Verification items for this drawing (mm, ordinates from the low corner). A direction names the side the tool comes from. Coordinates: 2 decimals unless noted, no trailing zeros. Order: outer loops, then holes, each group sorted by start corner. A loop starts at its lowest first (then second) coordinate and runs counter-clockwise, first axis right, second up. Notation, with made-up numbers: (-23, -17) -> (29, -17) arc R20 cw to (29, -10) -> close; hole circle Ø10 at (62.5, 56). An arc over 180 degrees is marked (long way). Write item = value, one per line. Start each with the question number.
1. Cross-section at B-B on x = 13.5. Record the cut outline in (y, z).
2. Release check for a two-part mould opening along X. For the marked faces 1, 2 and 3 record: +X half, -X half, draft (parallel to the pull), parting line (faces both ways), or undercut.
3. Set-up check for the marked faces 4 and 5: record each of +Z, -Z, +X, -X, +Y, -Y from which the full face is reachable in a straight line by a thin tool's end or side.
4. Cross-section at A-A on z = 60. Record the cut outline in (x, y), plus the area to 3 significant figures.
5. Cross-section at C-C on y = 55.5. Record the cut outline in (x, z), plus the area to 3 significant figures.
6. Thickness scan on line 1 along X through (y, z) = (53.5, 53.5); line 2 along Z through (x, y) = (68, 52); line 3 along Z through (x, y) = (12.5, 24). Record the ranges inside material, lowest first. Write a range as from..to.
7. Cross-section at D-D on z = 51. Record the cut outline in (x, y), plus the area to 3 significant figures.
8. Go/stop test with flat-tipped pins: P1, Ø1, axis at x = 78, z = 47.5, coming from the -Y side; P2, Ø5, axis at x = 14, y = 19.5, coming from the -Z side; P3, Ø9, axis at x = 43, y = 45.5, coming from the +Z side; P4, Ø1.5, axis at x = 23, y = 38, coming from the +Z side. Record where each tip stops, or that it passes through.
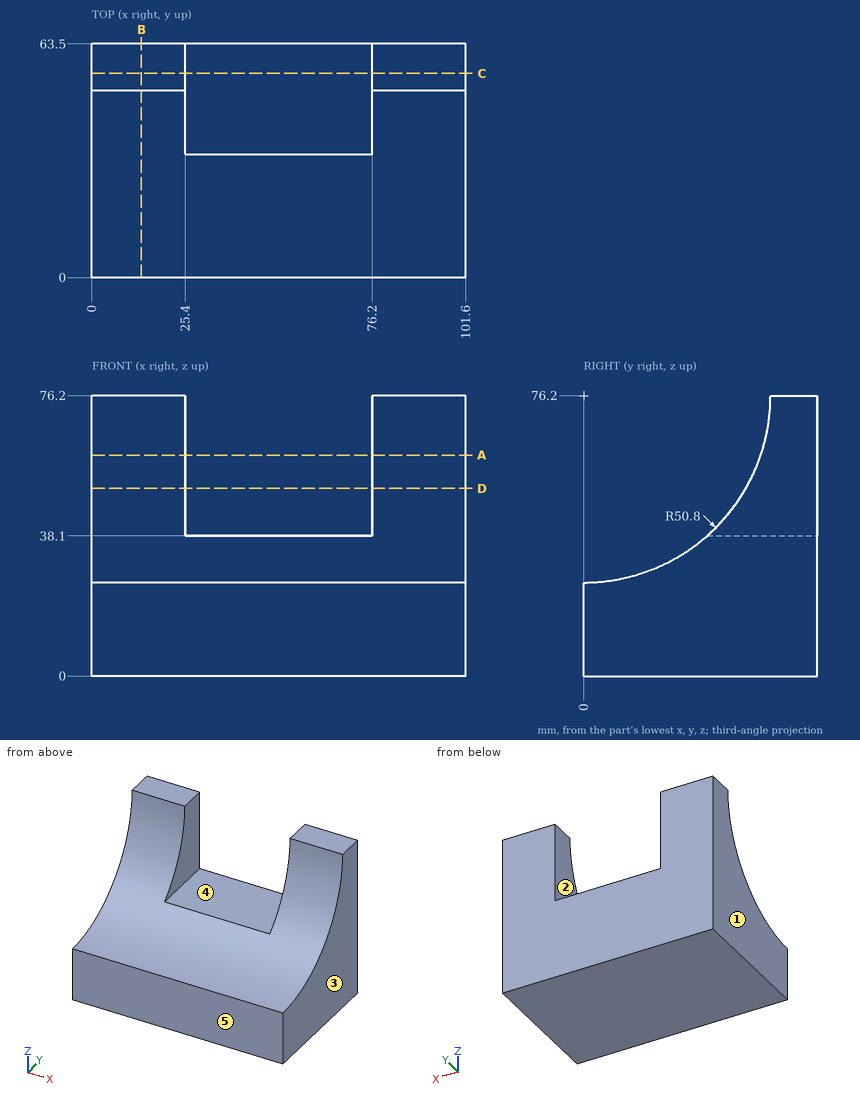
Worked out:
q1.outline = (0, 0) -> (63.5, 0) -> (63.5, 76.2) -> (50.8, 76.2) arc R50.8 cw to (0, 25.4) -> close
q2.face_1 = -X half
q2.face_2 = undercut
q2.face_3 = +X half
q3.face_4 = +Z, +Y, -Y
q3.face_5 = +Z, -Z, +X, -X, -Y
q4.outline = (0, 48.15) -> (25.4, 48.15) -> (25.4, 63.5) -> (0, 63.5) -> close; (76.2, 48.15) -> (101.6, 48.15) -> (101.6, 63.5) -> (76.2, 63.5) -> close
q4.area = 780 mm²
q5.outline = (0, 0) -> (101.6, 0) -> (101.6, 76.2) -> (76.2, 76.2) -> (76.2, 38.1) -> (25.4, 38.1) -> (25.4, 76.2) -> (0, 76.2) -> close
q5.area = 5,810 mm²
q6.line_1 = 0..25.4, 76.2..101.6
q6.line_2 = 0..38.1
q6.line_3 = 0..31.43
q7.outline = (0, 44.11) -> (25.4, 44.11) -> (25.4, 63.5) -> (0, 63.5) -> close; (76.2, 44.11) -> (101.6, 44.11) -> (101.6, 63.5) -> (76.2, 63.5) -> close
q7.area = 985 mm²
q8.P1 = 41.57
q8.P2 = 0
q8.P3 = 38.1
q8.P4 = 43.35
